```python
from build123d import *

# Parameters (mm, degrees)
BOSS_EXTRUDE1_DEPTH   = 6.35
SKETCH2_W             = 50.8
SKETCH2_H             = 25.4
CUT_EXTRUDE1_DEPTH    = 86.430512699
SKETCH5_R             = 7.9375
SKETCH5_R_2           = 2.0828
CUT_EXTRUDE4_DEPTH    = 86.430512699
SKETCH4_R             = 3.175
CUT_EXTRUDE5_DEPTH    = 86.430512699
SKETCH6_W             = 6.35
SKETCH6_H             = 6.604
BOSS_EXTRUDE2_DEPTH   = 3.81
CUT_EXTRUDE7_REACH    = 87.431
SKETCH8_R             = 3.6195
F_6_CLEARANCE_HOLE1_D = 3.5052


with BuildPart() as part:
    # Sketch1 → Boss-Extrude1 (new body)
    with BuildSketch(Plane.XY):
        with BuildLine():
            Line((-38.1, -38.1), (38.1, -38.1))
            ThreePointArc((38.1, -38.1), (76.2, 0), (38.1, 38.1))
            Line((38.1, 38.1), (-38.1, 38.1))
            Line((-38.1, 38.1), (-38.1, -38.1))
        make_face()
    extrude(amount=BOSS_EXTRUDE1_DEPTH)

    # Sketch2 → Cut-Extrude1 (cut, through all)
    with BuildSketch(Plane.XY.offset(6.35)):
        with Locations((-12.7, 0)):
            Rectangle(SKETCH2_W, SKETCH2_H)
    extrude(amount=-CUT_EXTRUDE1_DEPTH, mode=Mode.SUBTRACT)

    # Sketch5 → Cut-Extrude4 (cut, through all)
    with BuildSketch(Plane.XY.offset(6.35)):
        with Locations((38.1, 0)):
            Circle(SKETCH5_R)
        with Locations((38.1, 11.8999)):
            Circle(SKETCH5_R_2)
        with Locations((38.1, -11.8999)):
            Circle(SKETCH5_R_2)
    extrude(amount=-CUT_EXTRUDE4_DEPTH, mode=Mode.SUBTRACT)

    # Sketch4 → Cut-Extrude5 (cut, through all)
    with BuildSketch(Plane.XY.offset(6.35)):
        with Locations((0, -25.4)):
            Circle(SKETCH4_R)
    cut_extrude5 = extrude(amount=-CUT_EXTRUDE5_DEPTH, mode=Mode.SUBTRACT)

    # Mirror3: Cut-Extrude5 across plane
    add(cut_extrude5.mirror(Plane.ZX), mode=Mode.SUBTRACT)

    # Sketch6 → Boss-Extrude2 (add)
    with BuildSketch(Plane.ZY.offset(-12.7)):
        with Locations((3.175, 0)):
            Rectangle(SKETCH6_W, SKETCH6_H)
    extrude(amount=BOSS_EXTRUDE2_DEPTH)

    # Sketch8 → Cut-Extrude7 (cut, up to next)
    with BuildSketch(Plane.XY.offset(6.35), mode=Mode.PRIVATE) as cut_extrude7_sk1:
        with Locations((58.42, 0)):
            Circle(SKETCH8_R)
    cut_extrude7_tool1 = extrude(cut_extrude7_sk1.sketch, amount=-CUT_EXTRUDE7_REACH, mode=Mode.PRIVATE) & part.part
    add(cut_extrude7_tool1.solids().sort_by_distance((58.42, 0, 6.35))[0], mode=Mode.SUBTRACT)

    # #6 Clearance Hole1 (through all)
    with Locations(Plane(origin=(0, 0, 0), x_dir=(-1, 0, 0), z_dir=(0, 0, -1))):
        with Locations((-58.42, 10.16), (-58.42, -10.16)):
            Hole(F_6_CLEARANCE_HOLE1_D / 2)


solid = part.part
```
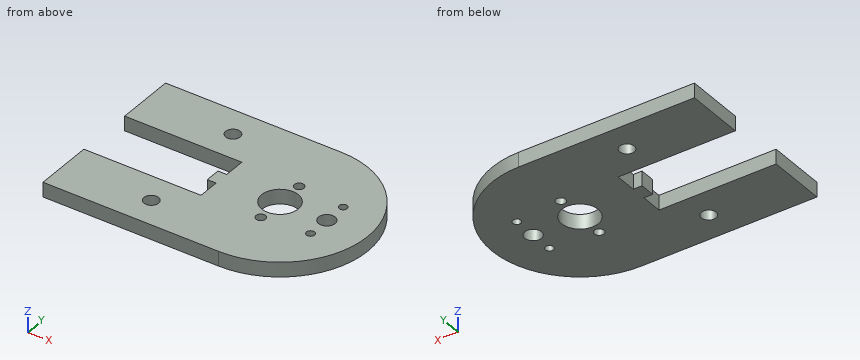
Read the model definition and answer for the solid it produces. Units are mm, in the model's axes. Give positions to 0.01 mm unless a question says otherwise; leave off trailing zeros. Write each loop counter-clockwise with the first axis right and the second up, starting at its lowest first coordinate (ties: lowest second). Pieces come first, ordered by that corner, then holes. Notation, with made-up numbers: (-22, 40.5) -> (14, 40.5) arc R28 cw to (14, 69.5) -> close; hole circle Ø8 at (-7.75, -3.5). An arc over 180 degrees is marked (long way). Answer as a JSON object with one key per item and string values.
1) Straight lines are drawn through the part: probe 1 along Y at (x, z) = (0, 2) (3 decimals); probe 2 along Y at (x, z) = (-25.5, 1); probe 3 along Y at (x, z) = (58.42, 3.5). For each, find the intervals that lie inside material, in ascending order. Write a range as from..to.
Findings below:
{"probe 1": "y = -38.1..-28.575, -22.225..-12.7, 12.7..22.225, 28.575..38.1", "probe 2": "y = -38.1..-12.7, 12.7..38.1", "probe 3": "y = -32.23..-11.91, -8.41..-3.62, 3.62..8.41, 11.91..32.23"}
2) Section B-B on y = 0 is taken. Write down the section's boundary in (x, z).
Findings below:
{"outline": "(8.89, 0) -> (30.16, 0) -> (30.16, 6.35) -> (8.89, 6.35) -> close; (46.04, 0) -> (54.8, 0) -> (54.8, 6.35) -> (46.04, 6.35) -> close; (62.04, 0) -> (76.2, 0) -> (76.2, 6.35) -> (62.04, 6.35) -> close"}
3) Flat-ended cylindrical pins translate along their axes: pin 1 Ø8.5 at (x, y) = (58.42, 0) entering from -Z; pin 2 Ø3 at (y, z) = (9, 3) entering from -X. Find the tip coordinate at first contact, or state that the pin passes through.
Findings below:
{"pin 1": "stops at z = 0", "pin 2": "stops at x = 12.7"}
4) Section A-A on x = -12.5 is taken. Write down the section's boundary in (y, z), then the cut area to 3 significant figures.
Findings below:
{"outline": "(-38.1, 0) -> (-12.7, 0) -> (-12.7, 6.35) -> (-38.1, 6.35) -> close; (12.7, 0) -> (38.1, 0) -> (38.1, 6.35) -> (12.7, 6.35) -> close", "area": "323 mm^2"}
5) Section C-C on z = 3 is taken. Count the separate pieces of the cut face and the enclosed holes in it, then the cut area to 3 significant figures.
Findings below:
{"separate pieces": "1", "enclosed holes": "8", "area": "6,470 mm^2"}
6) Section D-D on y = 25.4 is taken. Write down the section's boundary in (x, z) (3 decimals), then the cut area to 3 significant figures.
Findings below:
{"outline": "(-38.1, 0) -> (-3.175, 0) -> (-3.175, 6.35) -> (-38.1, 6.35) -> close; (3.175, 0) -> (66.498, 0) -> (66.498, 6.35) -> (3.175, 6.35) -> close", "area": "624 mm^2"}
